```python
from build123d import *

# Parameters (mm, degrees)
SKETCH1_R           = 1.5
BOSS_EXTRUDE1_DEPTH = 2
SKETCH2_W           = 34.7
SKETCH2_H           = 30
CUT_EXTRUDE1_DEPTH  = 10


with BuildPart() as part:
    # Sketch1 → Boss-Extrude1 (new body)
    with BuildSketch(Plane(origin=(0, 0, 0), x_dir=(1, 0, 0), z_dir=(0, 1, 0))):
        Polygon((0, 0), (2, 0), (2, 5), (4, 5), (4, 0), (10, 0), (10, 5), (12, 5), (12, 0), (72.4, 0), (72.4, 5), (74.4, 5), (74.4, 0), (80.4, 0), (80.4, 5), (82.4, 5), (82.4, 0), (84.4, 0), (84.4, 45), (82.4, 45), (82.4, 40), (80.4, 40), (80.4, 45), (74.4, 45), (74.4, 40), (72.4, 40), (72.4, 45), (12, 45), (12, 40), (10, 40), (10, 45), (4, 45), (4, 40), (2, 40), (2, 45), (0, 45), align=None)
        with Locations(Location((7, 42.5, 0), (0, 0, 270))):
            Circle(SKETCH1_R, mode=Mode.SUBTRACT)
        with Locations(Location((77.4, 42.5, 0), (0, 0, 90))):
            Circle(SKETCH1_R, mode=Mode.SUBTRACT)
        with Locations(Location((7, 2.5, 0), (0, 0, 90))):
            Circle(SKETCH1_R, mode=Mode.SUBTRACT)
        with Locations(Location((77.4, 2.5, 0), (0, 0, 270))):
            Circle(SKETCH1_R, mode=Mode.SUBTRACT)
    extrude(amount=BOSS_EXTRUDE1_DEPTH)

    # Sketch2 → Cut-Extrude1 (cut)
    with BuildSketch(Plane(origin=(0, 2, 0), x_dir=(1, 0, 0), z_dir=(0, 1, 0))):
        with Locations((42.2, 22.5)):
            Rectangle(SKETCH2_W, SKETCH2_H)
    extrude(amount=-CUT_EXTRUDE1_DEPTH, mode=Mode.SUBTRACT)


solid = part.part
```
Can you work these out from the model? Positions are in its coordinate system, mm. A direction names the side the tool comes from. Coordinates: 2 decimals unless noted, no trailing zeros. Write each loop counter-clockwise with the first axis right and the second up, starting at its lowest first coordinate (ties: lowest second). Pieces come first, ordered by that corner, then holes. Notation, with made-up numbers: M 5,66.5 L 47,66.5 A25 cw 47,87.5 Z; hole C 35,-4 d6. An arc over 180 degrees is marked long. Write item = value, one per line. Start each with the question number.
Q1. If we section it at D-D, the plane y = 1.65: State how many separate pieces and enclosed holes the cut face has, then the cut area to 3 significant figures.
Q2. If I drill on L1, parallel to Z at x = 77.4, y = 1.05; L2, parallel to X at y = 0.6, z = -10.5; L3, parallel to X at y = 1, z = -40.5, over which ranges is the centre line in solid material (lowest first)? Write a range as [from, to].
Q3. If we section it at B-B, the plane x = 7: Write out the boundary of the cut face in (y, z).
Q4. Thinking about a two-plate mould opening in Z: for faces 1 (the face through (11, 1, -5)), 2 (the face through (4, 1, -3)), 3 (the face through (78.3, 1, -41.3)), which applies, released by +Z, released by -Z, zero draft, split by the parting line, or undercut?
Q5. I'm going to push flat-ended pins straight in: pin 1 (1.8 mm diameter, centred on x = 7, z = -2.5, fed in from -Y); pin 2 (1 mm diameter, centred on x = 3, y = 1.5, fed in from +Z); pin 3 (0.6 mm diameter, centred on x = 10.5, y = 1, fed in from -Z). Where does each tip first touch, or does it pass through?
Q6. If we section it at A-A, the plane z = -12: Write out the boundary of the cut face in (x, y), then the cut area to 3 significant figures.
Q7. On a 3-axis mill with a long thin cutter (end or side, diameter ignored), from which of +Z, -Z, +X, -X, +Y, -Y can I reach the whole of each face in a straight line? I mean faces 4 (the face through (81, 1, -40)), 5 (the face through (1, 1, -45)), 6 (the face through (24.85, 1, -22)), 7 (the face through (3, 1, -5)). Say none if no direction works.
Q8. If we section it at C-C, the plane z = -42.5: Write out the boundary of the cut face in (x, y), then the cut area to 3 significant figures.
Check sheet entries:
q1.separate_pieces = 1
q1.enclosed_holes = 5
q1.area = 2,650 mm²
q2.L1 = [-45, -44], [-41, -4], [-1, 0]
q2.L2 = [0, 24.85], [59.55, 84.4]
q2.L3 = [0, 2], [4, 10], [12, 72.4], [74.4, 80.4], [82.4, 84.4]
q3.outline = M 0,-45 L 2,-45 L 2,-44 L 0,-44 Z; M 0,-41 L 2,-41 L 2,-4 L 0,-4 Z; M 0,-1 L 2,-1 L 2,0 L 0,0 Z
q4.face_1 = released by +Z
q4.face_2 = zero draft
q4.face_3 = undercut
q5.pin_1 = through
q5.pin_2 = -5
q5.pin_3 = -40
q6.outline = M 0,0 L 24.85,0 L 24.85,2 L 0,2 Z; M 59.55,0 L 84.4,0 L 84.4,2 L 59.55,2 Z
q6.area = 99.4 mm²
q7.face_4 = -Z, +Y, -Y
q7.face_5 = -Z, +X, -X, +Y, -Y
q7.face_6 = +Y, -Y
q7.face_7 = +Z, +Y, -Y
q8.outline = M 0,0 L 2,0 L 2,2 L 0,2 Z; M 4,0 L 5.5,0 L 5.5,2 L 4,2 Z; M 8.5,0 L 10,0 L 10,2 L 8.5,2 Z; M 12,0 L 72.4,0 L 72.4,2 L 12,2 Z; M 74.4,0 L 75.9,0 L 75.9,2 L 74.4,2 Z; M 78.9,0 L 80.4,0 L 80.4,2 L 78.9,2 Z; M 82.4,0 L 84.4,0 L 84.4,2 L 82.4,2 Z
q8.area = 141 mm²
